Read the model definition and answer for the solid it produces. Units are mm, in the model's axes. A direction names the side the tool comes from. Give positions to 0.01 mm unless a question says otherwise; leave off trailing zeros. Order: outer loops, then holes, each group sorted by start corner. A loop starts at its lowest first (then second) coordinate and runs counter-clockwise, first axis right, second up. Notation, with made-up numbers: M -39,13 L -22,13 A17 ccw -22,20 Z; hole C 66,12.5 d4. An arc over 180 degrees is marked long. Write item = value, one per line. Start each with the question number.
from build123d import *

# Parameters (mm, degrees)
CONG_1_R                = 0.5
ESQUISSE2_R             = 1.5
ENL_V_MAT_EXTRU_1_DEPTH = 10


with BuildPart() as part:
    # Esquisse1 → Révolution1 (revolve)
    with BuildSketch(Plane.XY, mode=Mode.PRIVATE) as r_volution1_sk:
        with BuildLine():
            Line((0, 5.7), (6.85, 5.7))
            Line((6.85, 5.7), (6.85, 3.7))
            Line((6.85, 3.7), (9.5, 0))
            Line((9.5, 0), (15.6, 0))
            Line((15.6, 0), (15.6, -2))
            Line((15.6, -2), (10, -2))
            ThreePointArc((10, -2), (8.212627426, -6.045887094), (4.880340938, -8.954455446))
            ThreePointArc((4.880340938, -8.954455446), (2.707365275, -10.683176126), (0, -11.3))
            Line((0, -11.3), (0, 5.7))
        make_face()
    revolve(r_volution1_sk.sketch.rotate(Axis((0, 5.7, 0), (0, -1, 0)), 90), axis=Axis((0, 5.7, 0), (0, -1, 0)))

    # Congé1
    cong_1_edges = [part.edges().sort_by_distance(p)[0] for p in [
        (0, 5.7, -6.85),
        (0, 0, -15.6),
        (0, -2, -15.6),
    ]]
    fillet(cong_1_edges, radius=CONG_1_R)

    # Esquisse2 → Enlèv. mat.-Extru.1 (cut)
    with BuildSketch(Plane(origin=(0, 0, 0), x_dir=(1, 0, 0), z_dir=(0, 1, 0))):
        with Locations(Location((0, 12.990381057, 0), (0, 0, 270))):
            Circle(ESQUISSE2_R)
        with Locations(Location((11.25, -6.495190528, 0), (0, 0, 270))):
            Circle(ESQUISSE2_R)
        with Locations(Location((-11.25, -6.495190528, 0), (0, 0, 270))):
            Circle(ESQUISSE2_R)
    extrude(amount=-ENL_V_MAT_EXTRU_1_DEPTH, mode=Mode.SUBTRACT)


solid = part.part
1) For faces 1 (the face through (-10.54, -1.01, -11.5)), 2 (the face through (-4.63, 4.44, -5.05)), determine the directions among +Z, -Z, +X, -X, +Y, -Y from which every point of the face is accessible in a straight line to the end or side of a thin tool.
2) For a pull along X with two mould halves and no side action, classify faces 3 (the face through (10, -2, 3)), 4 (the face through (10.675, -0.986, 7.881)), 5 (the face through (6.85, 3.47, -1.52)) as pulls with the +X half, pulls with the -X half, needs draft (parallel to the pull), parting line crosses it, or undercut.
3) Find section B-B on z = 0. Determine the outline of the cut face in (x, y).
4) Each of these flat-tipped pins is pushed along its axis until it touches: P1, Ø3.5, axis at x = 0, z = -12.99, coming from the -Y side; P2, Ø6, axis at y = -7.5, z = -6, coming from the -X side; P3, Ø4, axis at x = -3, z = 11, coming from the -Y side. Where does it stop, or does it pass through?
5) Find section C-C on y = -6.5. Determine the outline of the cut face in (x, z), plus the area to 3 significant figures.
6) Find section D-D on y = -4.75. Determine the outline of the cut face in (x, z), plus the area to 3 significant figures.
7) Find section A-A on x = 0. Determine the outline of the cut face in (y, z).
8) Find the intervals of material crossed by probe 1 along Y at (x, z) = (8.5, -7); probe 2 along Y at (x, z) = (1.5, -2.5); probe 3 along X at (y, z) = (3, 0.5), in increasing order. Write a range as [from, to].
Numbers:
q1.face_1 = +Y, -Y
q1.face_2 = +Y
q2.face_3 = needs draft
q2.face_4 = undercut
q2.face_5 = parting line crosses it
q3.outline = M -15.6,-1.5 A0.5 ccw -15.1,-2 L -10,-2 A10.2 ccw -4.88,-8.95 A6.25 ccw 4.88,-8.95 A10.2 ccw 10,-2 L 15.1,-2 A0.5 ccw 15.6,-1.5 L 15.6,-0.5 A0.5 ccw 15.1,0 L 9.5,0 L 6.85,3.7 L 6.85,5.2 A0.5 ccw 6.35,5.7 L -6.35,5.7 A0.5 ccw -6.85,5.2 L -6.85,3.7 L -9.5,0 L -15.1,0 A0.5 ccw -15.6,-0.5 Z
q4.P1 = -2
q4.P2 = -7.77
q4.P3 = -3.95
q5.outline = C 0,0 d15.72
q5.area = 194 mm2
q6.outline = C 0,0 d18.05
q6.area = 256 mm2
q7.outline = M -8.95,-4.88 A10.2 ccw -2,-10 L -2,-11.49 L 0,-11.49 L 0,-9.5 L 3.7,-6.85 L 5.2,-6.85 A0.5 ccw 5.7,-6.35 L 5.7,6.35 A0.5 ccw 5.2,6.85 L 3.7,6.85 L 0,9.5 L 0,15.1 A0.5 ccw -0.5,15.6 L -1.5,15.6 A0.5 ccw -2,15.1 L -2,10 A10.2 ccw -8.95,4.88 A6.25 ccw Z; M -2,-15.1 A0.5 ccw -1.5,-15.6 L -0.5,-15.6 A0.5 ccw 0,-15.1 L 0,-14.49 L -2,-14.49 Z
q8.probe_1 = [-2, 0]
q8.probe_2 = [-10.58, 5.7]
q8.probe_3 = [-7.33, 7.33]
